Autodesk Inventor part; units mm, degrees
ref_plane "YZ Plane" through (0, 0, 0) normal (1, 0, 0) x (0, 1, 0)
ref_plane "XZ Plane" through (0, 0, 0) normal (0, 1, 0) x (-1, 0, 0)
ref_plane "XY Plane" through (0, 0, 0) normal (0, 0, 1) x (1, 0, 0)
sketch "Skizze1" plane through (0, 0, 0) normal (0, 0, 1) x (1, 0, 0)
  line L0 (-26, -30) -> (26, -30)
  line L1 (30, -26) -> (30, 26)
  line L2 (26, 30) -> (-26, 30)
  line L3 (-30, 26) -> (-30, -26)
  line L4 (-30, -30) -> (30, 30) construction
  line L5 (30, -30) -> (-30, 30) construction
  arc A0 (30, 26) -> (26, 30) centre (26, 26) ccw
  arc A1 (26, -30) -> (30, -26) centre (26, -26) ccw
  arc A2 (-30, -26) -> (-26, -30) centre (-26, -26) ccw
  arc A3 (-26, 30) -> (-30, 26) centre (-26, 26) ccw
  point P0 (0, 0)
  dimension "d0" = 4
  dimension "d1" = 60
extrude "Extrusion1" add sketch "Skizze1" against normal blind 100
sketch "Skizze2" plane through (0, 0, 0) normal (0, 0, 1) x (1, 0, 0)
  circle A0 centre (0, 0) radius 19.05
  dimension "d4" = 38.1
extrude "Extrusion2" add sketch "Skizze2" along normal blind 1.6
sketch "Skizze4" plane through (0, 0, 0) normal (0, 0, 1) x (1, 0, 0)
  circle A0 centre (0, 0) radius 19.05
  line L0 (30, 26) -> (30, -26)
  arc A1 (30, 26) -> (26, 30) centre (26, 26) ccw
  line L1 (-26, 30) -> (26, 30)
  arc A2 (-26, 30) -> (-30, 26) centre (-26, 26) ccw
  line L2 (-30, -26) -> (-30, 26)
  arc A3 (-30, -26) -> (-26, -30) centre (-26, -26) ccw
  line L3 (26, -30) -> (-26, -30)
  arc A4 (26, -30) -> (30, -26) centre (26, -26) ccw
  line L4 (26, -26) -> (-26, 26) construction
  line L5 (-23.57, 23.57) -> (23.57, 23.57) construction
  line L6 (23.57, 23.57) -> (23.57, -23.57) construction
  line L7 (23.57, -23.57) -> (-23.57, -23.57) construction
  line L8 (-23.57, -23.57) -> (-23.57, 23.57) construction
  line L9 (-23.57, 23.57) -> (23.57, -23.57) construction
  line L10 (23.57, 23.57) -> (-23.57, -23.57) construction
  dimension "d15" = 47.14
hole "Bohrung1" at (23.57, 23.57, 0) at (-23.57, 23.57, 0) at (-23.57, -23.57, 0) at (23.57, -23.57, 0) direction (0, 0, -1) diameter 4.5 end through all
sketch "Skizze5" plane through (0, 0, 1.6) normal (0, 0, 1) x (1, 0, 0)
  circle A0 centre (0, 0) radius 4
  dimension "d23" = 8
extrude "Extrusion4" add sketch "Skizze5" along normal blind 22.4
sketch "Skizze7" plane through (0, 0, -100) normal (0, 0, -1) x (-1, 0, 0)
  circle A0 centre (23.57, -23.57) radius 2.25
  circle A1 centre (-23.57, 23.57) radius 2.25
  circle A2 centre (23.57, 23.57) radius 2.25
  circle A3 centre (-23.57, -23.57) radius 2.25
  line L0 (-30, 26) -> (-30, -26)
  arc A4 (-30, -26) -> (-26, -30) centre (-26, -26) ccw
  line L1 (-26, -30) -> (26, -30)
  arc A5 (26, -30) -> (30, -26) centre (26, -26) ccw
  line L2 (30, -26) -> (30, 26)
  arc A6 (30, 26) -> (26, 30) centre (26, 26) ccw
  line L3 (26, 30) -> (-26, 30)
  arc A7 (-26, 30) -> (-30, 26) centre (-26, 26) ccw
  circle A8 centre (23.57, -23.57) radius 6.43 construction
  line L4 (30, -26) -> (30, 26)
  line L5 (30, -17.14) -> (23.57, -17.14)
  line L6 (-26, -30) -> (26, -30)
  line L7 (17.14, -30) -> (17.14, -23.57)
  arc A9 (23.57, -17.14) -> (17.14, -23.57) centre (23.57, -23.57) ccw
  arc A10 (-17.14, -23.57) -> (-23.57, -17.14) centre (-23.57, -23.57) ccw
  arc A11 (17.2019, 24.4599) -> (23.57, 17.14) centre (23.57, 23.57) ccw
  arc A12 (-23.57, 17.14) -> (-17.14, 23.57) centre (-23.57, 23.57) ccw
  line L8 (23.57, 17.14) -> (30, 17.14)
  line L9 (17.14, 23.57) -> (17.14, 30)
  line L10 (26, 30) -> (-26, 30)
  line L11 (-17.14, 23.57) -> (-17.14, 30)
  line L12 (-23.57, 17.14) -> (-30, 17.14)
  line L13 (-23.57, -17.14) -> (-30, -17.14)
  line L14 (-17.14, -23.57) -> (-17.14, -30)
  point P0 (0, 0)
extrude "Extrusion6" cut sketch "Skizze7" against normal blind 93.2 contours A7 L3 L11 A12 L12 L0 | L13 A10 L14 L1 A4 L0 | L3 A6 L2 L8 A11 L9 | L7 A9 L5 L2 A5 L1
sketch "Skizze8" plane through (0, 0, -100) normal (0, 0, -1) x (-1, 0, 0)
  circle A0 centre (23.57, -23.57) radius 2.25 construction
  circle A1 centre (-23.57, 23.57) radius 2.25 construction
  circle A2 centre (23.57, 23.57) radius 2.25 construction
  circle A3 centre (-23.57, -23.57) radius 2.25 construction
  circle A4 centre (0, 0) radius 19.05 construction
  line L0 (-30, 26) -> (-30, -26) construction
  arc A5 (-26, 30) -> (-30, 26) centre (-26, 26) ccw construction
  line L1 (26, 30) -> (-26, 30) construction
  arc A6 (30, 26) -> (26, 30) centre (26, 26) ccw construction
  line L2 (30, -26) -> (30, 26) construction
  arc A7 (26, -30) -> (30, -26) centre (26, -26) ccw construction
  line L3 (-26, -30) -> (26, -30) construction
  arc A8 (-30, -26) -> (-26, -30) centre (-26, -26) ccw construction
  circle A9 centre (0, 0) radius 42.4264 construction
  line L4 (30, 30) -> (-30, 30) construction
  line L5 (-30, 30) -> (-30, -30) construction
  line L6 (-30, -30) -> (30, -30) construction
  line L7 (30, -30) -> (30, 30) construction
  line L8 (30, 30) -> (-30, -30) construction
  line L9 (-30, 30) -> (30, -30) construction
  line L10 (-17.14, -30) -> (17.14, -30) construction
  line L11 (-30, 17.14) -> (-30, -17.14) construction
sketch "Skizze9" plane through (0, 0, -100) normal (0, 0, -1) x (-1, 0, 0)
  circle A0 centre (0, 0) radius 4
extrude "Extrusion7" add sketch "Skizze9" along normal blind 15
chamfer "Fase1" distance 0.5 angle 45 2 edges at (4, 0, -115) (-4, 0, 24)
equation "\"d1\" = breite"
equation "\"d2\" = Laenge"
equation "\"d4\" = fit"
equation "\"d5\" = fit_l"
equation "\"d15\" = lochabstand"
equation "\"d16\" = bohrung_d"
equation "\"d23\" = schaft_d"
equation "\"d24\" = schaft_l"
equation "\"d28\" = Laenge - Mount_l"
equation "\"breite\" = 60"
equation "\"lochabstand\" = 47.14"
equation "\"schaft_d\" = 8"
equation "\"fit\" = 38.1"
equation "\"fit_l\" = 1.6"
equation "\"Mount_l\" = 6.8"
equation "\"Laenge\" = 100"
equation "\"bohrung_d\" = 4.5"
properties part number "Nema24 - L100" material "Stahl"
Could you check a few things on this model? Use its own coordinates, in mm. A direction names the side the tool comes from. Coordinates: 2 decimals unless noted, no trailing zeros. Write each loop counter-clockwise with the first axis right and the second up, starting at its lowest first coordinate (ties: lowest second). Pieces come first, ordered by that corner, then holes. Notation, with made-up numbers: M 62.25,63.25 L 84.25,63.25 A28 cw 84.25,101.25 Z; hole C 57,84.5 d8. An arc over 180 degrees is marked long. Answer as CSV lines item,"result". Start each with the question number.
1) For P1, Ø1.9, axis at x = -26.5, z = -52, coming from the +Y side; P2, Ø7, axis at x = 26.5, z = -32, coming from the +Y side; P3, Ø5, axis at x = 13, y = -10.5, coming from the -Z side, each with a flat end and sliding along its axis, tell me the tip position at first contact or that it passes through.
2) We'd pull the mould along X, two halves only. Please class faces 1 (the cylindrical face through (-0.867, 3.905, 12.397)), 2 (the flat face through (0, -30, -49)), 3 (the cylindrical face through (-25.467, 22.36, -3.448)), 4 (the cylindrical face through (-25.09, -21.91, -3.45)): +X half, -X half, draft (parallel to the pull), parting line (faces both ways), or undercut.
3) I want a section at A-A, the plane x = 0. Please give me the cut outline in (y, z), and give its area (3 significant figures).
4) I want a section at D-D, the plane y = 6.5. Please give me the cut outline in (x, z).
5) I want a section at C-C, the plane z = -18.5. Please give me the cut outline in (x, y).
6) For faces 5 (the flat face through (17.14, -27, -54)), 6 (the cylindrical face through (-15.12, 11.59, 0.79)), 7 (the flat face through (17.14, 27, -54)), 8 (the cylindrical face through (-19.074, -18.974, -54.052)), which set-ups out of +Z, -Z, +X, -X, +Y, -Y let a thin tool reach every point of the face, with its end or its side?
7) Please list where these lines run through material, in increasing order: line 1 (Y direction, x = -23.57, z = -5); line 2 (X direction, y = -23, z = -3). Write a range as from..to.
Data:
1,P1,"stops at y = 17.14"
1,P2,"stops at y = 17.17"
1,P3,"stops at z = -100"
2,face 1,"parting line"
2,face 2,"draft"
2,face 3,"undercut"
2,face 4,"undercut"
3,outline,"M -30,-100 L -4,-100 L -4,-114.5 L -3.5,-115 L 3.5,-115 L 4,-114.5 L 4,-100 L 30,-100 L 30,0 L 19.05,0 L 19.05,1.6 L 4,1.6 L 4,23.5 L 3.5,24 L -3.5,24 L -4,23.5 L -4,1.6 L -19.05,1.6 L -19.05,0 L -30,0 Z"
3,area,"6,360 mm^2"
4,outline,"M -30,-100 L 30,-100 L 30,0 L 17.91,0 L 17.91,1.6 L -17.91,1.6 L -17.91,0 L -30,0 Z"
5,outline,"M -30,-17.14 L -23.57,-17.14 A6.43 cw -17.14,-23.57 L -17.14,-30 L 17.14,-30 L 17.14,-23.57 A6.43 cw 23.57,-17.14 L 30,-17.14 L 30,17.14 L 23.57,17.14 A6.43 cw 17.14,23.57 L 17.14,30 L -17.14,30 L -17.14,23.57 A6.43 cw -23.57,17.14 L -30,17.14 Z"
6,face 5,"-Z, +X, -Y"
6,face 6,"+Z"
6,face 7,"-Z, +X, +Y"
6,face 8,"-Z, -X, -Y"
7,line 1,"y = -30..-25.82, -21.32..21.32, 25.82..30"
7,line 2,"x = -30..-25.75, -21.39..21.39, 25.75..30"
